Geometry check sheet. Reference: the model listing, model coordinates, mm. Face numbers are marked on the shaded views. Give positions to 0.01 mm unless a question says otherwise; leave off trailing zeros. Write each loop counter-clockwise with the first axis right and the second up, starting at its lowest first coordinate (ties: lowest second). Pieces come first, ordered by that corner, then holes. Notation, with made-up numbers: (61.25, -20.75) -> (117.25, -20.75) arc R8 cw to (117.25, -8.75) -> close; hole circle Ø11 at (18, 14.5). An arc over 180 degrees is marked (long way). Use a Markdown table: item, result. Add a question column.
from build123d import *

# Parameters (mm, degrees)
PAD_DEPTH            = 5
SKETCH001_R          = 2.5
POCKET_DEPTH         = 288.500559
POCKET001_DEPTH      = 283.500559
POCKET001_DEPTH_BACK = 288.500559
SKETCH003_R          = 20
POCKET002_DEPTH      = 2.5
SKETCH004_R          = 4.5
POCKET003_DEPTH      = 288.500559
POCKET003_DEPTH_BACK = 283.500559


with BuildPart() as part:
    # Sketch → Pad (new body)
    with BuildSketch(Plane.XY):
        Polygon((0, 0), (0, 69), (32, 69), (32, -69), (0, -69), align=None)
    pad = extrude(amount=PAD_DEPTH)

    # Sketch001 → Pocket (cut, through all)
    with BuildSketch(Plane(origin=(23.5, 14.75, 0), x_dir=(1, 0, 0), z_dir=(0, 0, 1))):
        Circle(SKETCH001_R)
        with Locations((0, 47)):
            Circle(SKETCH001_R)
    pocket = extrude(amount=POCKET_DEPTH, mode=Mode.SUBTRACT)

    # Sketch002 → Pocket001 (cut, two sides)
    with BuildSketch(Plane(origin=(23, -1.25, 0), x_dir=(1, 0, 0), z_dir=(0, 0, 1))) as pocket001_sk:
        with BuildLine():
            ThreePointArc((3, 0), (0, 3), (-3, 0))
            Line((-3, 0), (-3, -14))
            ThreePointArc((-3, -14), (0, -17), (3, -14))
            Line((3, -14), (3, 0))
        make_face()
        with BuildLine():
            ThreePointArc((3, -46), (0, -43), (-3, -46))
            Line((-3, -46), (-3, -60))
            ThreePointArc((-3, -60), (0, -63), (3, -60))
            Line((3, -60), (3, -46))
        make_face()
    pocket001 = extrude(amount=-POCKET001_DEPTH, mode=Mode.SUBTRACT) + extrude(pocket001_sk.sketch, amount=POCKET001_DEPTH_BACK, mode=Mode.SUBTRACT)

    # Sketch003 → Pocket002 (cut)
    with BuildSketch(Plane(origin=(0, 38.25, 5), x_dir=(1, 0, 0), z_dir=(0, 0, 1))):
        Circle(SKETCH003_R)
    pocket002 = extrude(amount=-POCKET002_DEPTH, mode=Mode.SUBTRACT)

    # Sketch004 → Pocket003 (cut, two sides)
    with BuildSketch(Plane(origin=(0, 38.25, 5), x_dir=(1, 0, 0), z_dir=(0, 0, 1))) as pocket003_sk:
        Circle(SKETCH004_R)
    pocket003 = extrude(amount=-POCKET003_DEPTH, mode=Mode.SUBTRACT) + extrude(pocket003_sk.sketch, amount=POCKET003_DEPTH_BACK, mode=Mode.SUBTRACT)

    # Mirrored: Pad, Pocket, Pocket001, Pocket002, Pocket003 across Sketch V_Axis
    add(pad.mirror(Plane(origin=(0, 0, 0), x_dir=(0, 0, 1), z_dir=(1, 0, 0))))
    add(pocket.mirror(Plane(origin=(0, 0, 0), x_dir=(0, 0, 1), z_dir=(1, 0, 0))), mode=Mode.SUBTRACT)
    add(pocket001.mirror(Plane(origin=(0, 0, 0), x_dir=(0, 0, 1), z_dir=(1, 0, 0))), mode=Mode.SUBTRACT)
    add(pocket002.mirror(Plane(origin=(0, 0, 0), x_dir=(0, 0, 1), z_dir=(1, 0, 0))), mode=Mode.SUBTRACT)
    add(pocket003.mirror(Plane(origin=(0, 0, 0), x_dir=(0, 0, 1), z_dir=(1, 0, 0))), mode=Mode.SUBTRACT)


solid = part.part
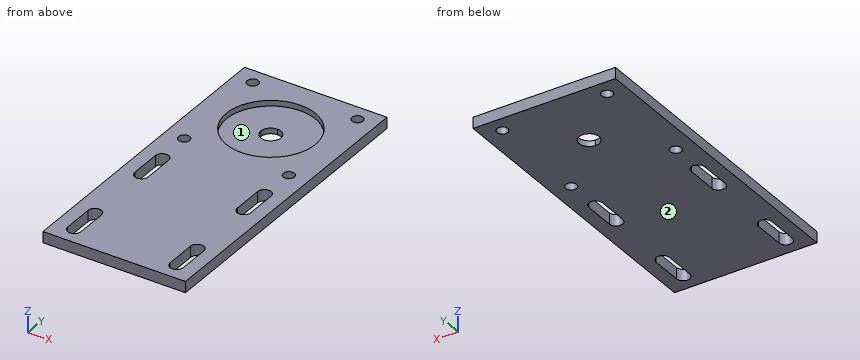
1) Sectioned sample at D-D, the plane x = -23.5. Enter the section's corners in (y, z), and give its area (3 significant figures).
2) Sectioned sample at B-B, the plane y = 14.75. Enter the section's corners in (x, z).
3) Sectioned sample at A-A, the plane z = 3.25. Count the separate pieces of the cut face and the enclosed holes in it, and give its area (3 significant figures).
4) Draft check along X on the marked faces 1 and 2. Enter one of: +X half, -X half, draft (parallel to the pull), parting line (faces both ways), or undercut.
5) Gauge pin test, flat ends, axial feed: P1, Ø6, axis at x = 8, y = -25, coming from the -Z side; P2, Ø12, axis at x = 3, y = 43, coming from the +Z side. Record the tip position at first contact, or that the pin passes through.
6) Material ranges on probe 1 along X at (y, z) = (38.25, 4.45); probe 2 along X at (y, z) = (-0.5, 2.7); probe 3 along Y at (x, z) = (-0.5, 3.65), recorded low to high. Write a range as [from, to].
7) Sectioned sample at C-C, the plane x = 23. Enter the section's corners in (y, z), and give its area (3 significant figures).
Check values:
| question | item | result |
|---|---|---|
| 1 | outline | (-69, 0) -> (-64.21, 0) -> (-64.21, 5) -> (-69, 5) -> close; (-44.29, 0) -> (-18.21, 0) -> (-18.21, 5) -> (-44.29, 5) -> close; (1.71, 0) -> (12.25, 0) -> (12.25, 5) -> (1.71, 5) -> close; (17.25, 0) -> (59.25, 0) -> (59.25, 5) -> (17.25, 5) -> close; (64.25, 0) -> (69, 0) -> (69, 5) -> (64.25, 5) -> close |
| 1 | area | 441 mm² |
| 2 | outline | (-32, 0) -> (-26, 0) -> (-26, 5) -> (-32, 5) -> close; (-21, 0) -> (21, 0) -> (21, 5) -> (-21, 5) -> close; (26, 0) -> (32, 0) -> (32, 5) -> (26, 5) -> close |
| 3 | separate pieces | 1 |
| 3 | enclosed holes | 9 |
| 3 | area | 7,050 mm² |
| 4 | face 1 | undercut |
| 4 | face 2 | draft |
| 5 | P1 | z = 0 |
| 5 | P2 | z = 2.5 |
| 6 | probe 1 | [-32, -20], [20, 32] |
| 6 | probe 2 | [-32, -25.9], [-20.1, 20.1], [25.9, 32] |
| 6 | probe 3 | [-69, 18.26], [58.24, 69] |
| 7 | outline | (-69, 0) -> (-64.25, 0) -> (-64.25, 5) -> (-69, 5) -> close; (-44.25, 0) -> (-18.25, 0) -> (-18.25, 5) -> (-44.25, 5) -> close; (1.75, 0) -> (12.3, 0) -> (12.3, 5) -> (1.75, 5) -> close; (17.2, 0) -> (59.3, 0) -> (59.3, 5) -> (17.2, 5) -> close; (64.2, 0) -> (69, 0) -> (69, 5) -> (64.2, 5) -> close |
| 7 | area | 441 mm² |
